Build history of the part. All positions in model axes, mm. Coordinates: 2 decimals unless noted, no trailing zeros. Order: outer loops, then holes, each group sorted by start corner. A loop starts at its lowest first (then second) coordinate and runs counter-clockwise, first axis right, second up. Notation, with made-up numbers: (-7.75, -23) - (19.25, -23) arc R24 cw to (19.25, -4) - close; hole circle Ø5 at (-21, -6). An arc over 180 degrees is marked (long way). Return JSON: item names as keys, results as strings.
from build123d import *

# Parameters (mm, degrees)
SKETCH1_W           = 220
SKETCH1_H           = 220
BOSS_EXTRUDE1_DEPTH = 4.5
CUT_EXTRUDE1_REACH  = 6.5
SKETCH2_R           = 13
CUT_EXTRUDE2_REACH  = 6.5
SKETCH3_R           = 2.5
CUT_EXTRUDE3_REACH  = 6.5
SKETCH4_R           = 2.5


with BuildPart() as part:
    # Sketch1 → Boss-Extrude1 (new body)
    with BuildSketch(Plane(origin=(0, 0, 0), x_dir=(1, 0, 0), z_dir=(0, 1, 0))):
        Rectangle(SKETCH1_W, SKETCH1_H)
    extrude(amount=BOSS_EXTRUDE1_DEPTH)

    # Sketch2 → Cut-Extrude1 (cut, up to next)
    with BuildSketch(Plane(origin=(0, 4.5, 0), x_dir=(1, 0, 0), z_dir=(0, 1, 0)), mode=Mode.PRIVATE) as cut_extrude1_sk1:
        with Locations((20, -53.431457505)):
            Circle(SKETCH2_R)
    cut_extrude1_tool1 = extrude(cut_extrude1_sk1.sketch, amount=-CUT_EXTRUDE1_REACH, mode=Mode.PRIVATE) & part.part
    add(cut_extrude1_tool1.solids().sort_by_distance((20, 4.5, 53.431458))[0], mode=Mode.SUBTRACT)

    # Sketch3 → Cut-Extrude2 (cut, up to next)
    with BuildSketch(Plane(origin=(0, 4.5, 0), x_dir=(1, 0, 0), z_dir=(0, 1, 0)), mode=Mode.PRIVATE) as cut_extrude2_sk1:
        with Locations((95, -93)):
            Circle(SKETCH3_R)
    cut_extrude2_tool1 = extrude(cut_extrude2_sk1.sketch, amount=-CUT_EXTRUDE2_REACH, mode=Mode.PRIVATE) & part.part
    add(cut_extrude2_tool1.solids().sort_by_distance((95, 4.5, 93))[0], mode=Mode.SUBTRACT)
    # Sketch3 → Cut-Extrude2 (cut, up to next)
    with BuildSketch(Plane(origin=(0, 4.5, 0), x_dir=(1, 0, 0), z_dir=(0, 1, 0)), mode=Mode.PRIVATE) as cut_extrude2_sk2:
        with Locations((-70, -93)):
            Circle(SKETCH3_R)
    cut_extrude2_tool2 = extrude(cut_extrude2_sk2.sketch, amount=-CUT_EXTRUDE2_REACH, mode=Mode.PRIVATE) & part.part
    add(cut_extrude2_tool2.solids().sort_by_distance((-70, 4.5, 93))[0], mode=Mode.SUBTRACT)

    # Sketch4 → Cut-Extrude3 (cut, up to next)
    with BuildSketch(Plane(origin=(0, 0, 0), x_dir=(-1, 0, 0), z_dir=(0, -1, 0)), mode=Mode.PRIVATE) as cut_extrude3_sk1:
        with Locations((-60, 96)):
            Circle(SKETCH4_R)
    cut_extrude3_tool1 = extrude(cut_extrude3_sk1.sketch, amount=-CUT_EXTRUDE3_REACH, mode=Mode.PRIVATE) & part.part
    add(cut_extrude3_tool1.solids().sort_by_distance((60, 0, -96))[0], mode=Mode.SUBTRACT)
    # Sketch4 → Cut-Extrude3 (cut, up to next)
    with BuildSketch(Plane(origin=(0, 0, 0), x_dir=(-1, 0, 0), z_dir=(0, -1, 0)), mode=Mode.PRIVATE) as cut_extrude3_sk2:
        with Locations((60, 96)):
            Circle(SKETCH4_R)
    cut_extrude3_tool2 = extrude(cut_extrude3_sk2.sketch, amount=-CUT_EXTRUDE3_REACH, mode=Mode.PRIVATE) & part.part
    add(cut_extrude3_tool2.solids().sort_by_distance((-60, 0, -96))[0], mode=Mode.SUBTRACT)


solid = part.part
1. Cut at A-A on z = 93. Give the cut face in (x, y).
Check values:
{"outline": "(-110, 0) - (-72.5, 0) - (-72.5, 4.5) - (-110, 4.5) - close; (-67.5, 0) - (92.5, 0) - (92.5, 4.5) - (-67.5, 4.5) - close; (97.5, 0) - (110, 0) - (110, 4.5) - (97.5, 4.5) - close"}
2. Mould opens along X. For faces 1 (the cylindrical face through (94.67, 2.28, 90.52)), 2 (the flat face through (-2, 4.5, -2)) say: pulls with the +X half, pulls with the -X half, needs draft (parallel to the pull), parting line crosses it, or undercut.
Check values:
{"face 1": "undercut", "face 2": "needs draft"}
3. Drop a flat-ended pin along its axis: pin 1 (8 mm diameter, centred on x = -70, z = 93, fed in from +Y). Give the stop position or say it passes through.
Check values:
{"pin 1": "y = 4.5"}
4. Probe L1, parallel to X at y = 2.3, z = -96; L2, parallel to X at y = 2.8, z = 93; L3, parallel to Z at x = 20.5, y = 1.7. List the from-to ranges inside material, lowest first.
Check values:
{"L1": "-110 to -62.5, -57.5 to 57.5, 62.5 to 110", "L2": "-110 to -72.5, -67.5 to 92.5, 97.5 to 110", "L3": "-110 to 40.44, 66.42 to 110"}
5. Cut at B-B on x = 60. Give the cut face in (y, z).
Check values:
{"outline": "(0, -110) - (4.5, -110) - (4.5, -98.5) - (0, -98.5) - close; (0, -93.5) - (4.5, -93.5) - (4.5, 110) - (0, 110) - close"}
6. Cut at C-C on z = 45.5. Give the cut face in (x, y).
Check values:
{"outline": "(-110, 0) - (9.7, 0) - (9.7, 4.5) - (-110, 4.5) - close; (30.3, 0) - (110, 0) - (110, 4.5) - (30.3, 4.5) - close"}
